Check sheet for the drawn part. Datum: minimum x, y, z corner. Units: mm. A direction names the side the tool comes from. Give positions to 0.01 mm unless a question says otherwise; leave off trailing zeros. Write each loop counter-clockwise with the first axis right and the second up, starting at its lowest first coordinate (ties: lowest second). Pieces come first, ordered by that corner, then holes.
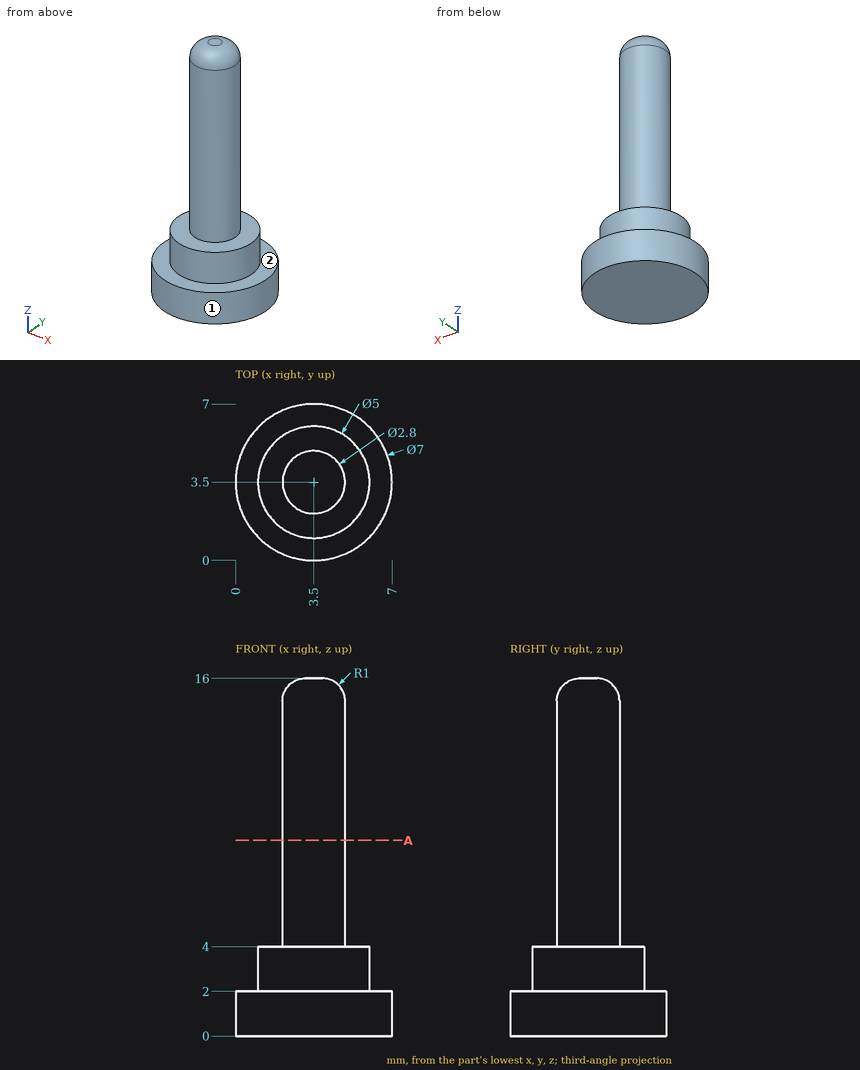
1) Sectioned sample at A-A on z = 8.75. Record the boundary of the cut face in (x, y), then the cut area to 3 significant figures.
2) Scan lines: L1, parallel to Z at x = 4.5, y = 5.25; L2, parallel to Z at x = 0.75, y = 5.5; L3, parallel to Y at x = 3.25, z = 10.25. Record each from-to range of solid material in increasing order.
3) Gauge pin test, flat ends, axial feed: pin 1 (1.5 mm diameter, centred on x = 2, z = 7, fed in from -Y); pin 2 (3 mm diameter, centred on x = 3.5, z = 8, fed in from +Y); pin 3 (4 mm diameter, centred on y = 5.5, z = 10, fed in from -X). Record the tip position at first contact, or that the pin passes through.
4) Access from +Z, -Z, +X, -X, +Y, -Y to the whole of each face (thin tool, end or side, straight path). Record for the marked faces 1 and 2.
Answers below:
1. outline: circle Ø2.8 at (3.5, 3.5)
1. area: 6.16 mm2
2. L1: z = 0 to 4
2. L2: z = 0 to 2
2. L3: y = 2.12 to 4.88
3. pin 1: stops at y = 2.32
3. pin 2: stops at y = 4.9
3. pin 3: stops at x = 2.1
4. face 1: +Z, -Z
4. face 2: +Z
